Input: part model. Units: mm. Frame: model coordinates. Face numbers are marked on the shaded views. A direction names the side the tool comes from. Round coordinates to 2 decimals unless told otherwise and drop trailing zeros. Order: outer loops, then holes, each group sorted by start corner. A loop starts at its lowest first (then second) coordinate and runs counter-clockwise, first axis right, second up. Notation, with made-up numbers: (-8.75, 23) - (40.25, 23) arc R27 ccw to (40.25, 53) - close; hole circle Ø3 at (-22.75, 46.25). An arc over 180 degrees is marked (long way). One line per item, written item: value. Start each with the question number.
from build123d import *

# Parameters (mm, degrees)
SKETCH_1_W          = 67
SKETCH_1_H          = 122
EXTRUDE_1_DEPTH     = 4
SKETCH_2_W          = 4
SKETCH_2_H          = 122
EXTRUDE_2_DEPTH     = 61
FILLET_1_R          = 2
SKETCH_4_R          = 38
SKETCH_4_R_2        = 2
CUT_EXTRUDE_1_DEPTH = 11
CUT_EXTRUDE_START   = -11
SKETCH_5_R          = 36
SKETCH_5_R_2        = 2
CUT_EXTRUDE_2_DEPTH = 11


with BuildPart() as part:
    # Эскиз1 → Бобышка-Вытянуть1 (new body)
    with BuildSketch(Plane(origin=(0, 0, 0), x_dir=(1, 0, 0), z_dir=(0, 1, 0))):
        Rectangle(SKETCH_1_W, SKETCH_1_H)
    extrude(amount=EXTRUDE_1_DEPTH)

    # Эскиз2 → Бобышка-Вытянуть2 (add)
    with BuildSketch(Plane(origin=(0, 4, 0), x_dir=(1, 0, 0), z_dir=(0, 1, 0))):
        with Locations((-31.5, 0)):
            Rectangle(SKETCH_2_W, SKETCH_2_H)
        with Locations((31.5, 0)):
            Rectangle(SKETCH_2_W, SKETCH_2_H)
    extrude(amount=EXTRUDE_2_DEPTH)

    # Скругление1
    fillet_1_edges = [part.edges().sort_by_distance(p)[0] for p in [
        (-29.5, 4, 0),
        (29.5, 4, 0),
        (33.5, 0, 0),
        (-33.5, 0, 0),
    ]]
    fillet(fillet_1_edges, radius=FILLET_1_R)

    # Эскиз4 → Вырез-Вытянуть1 (cut)
    with BuildSketch(Plane(origin=(33.5, 0, 0), x_dir=(0, 0, -1), z_dir=(1, 0, 0))):
        with Locations((0, 65)):
            Circle(SKETCH_4_R)
        with Locations((0, 12)):
            Circle(SKETCH_4_R_2)
        with Locations((-31.152618372, 22.122099298)):
            Circle(SKETCH_4_R_2)
        with Locations((-50.405995364, 48.622099298)):
            Circle(SKETCH_4_R_2)
        with Locations((50.405995364, 48.622099298)):
            Circle(SKETCH_4_R_2)
        with Locations((31.152618372, 22.122099298)):
            Circle(SKETCH_4_R_2)
    extrude(amount=-CUT_EXTRUDE_1_DEPTH, mode=Mode.SUBTRACT)

    # Эскиз5 → Вырез-Вытянуть2 (cut)
    with BuildSketch(Plane.ZY.offset(33.5).offset(CUT_EXTRUDE_START)):
        with Locations((0, 65)):
            Circle(SKETCH_5_R)
        with Locations(Location((0, 12, 0), (0, 0, 180))):
            Circle(SKETCH_5_R_2)
        with Locations(Location((-31.152618372, 22.122099298, 0), (0, 0, 180))):
            Circle(SKETCH_5_R_2)
        with Locations(Location((-50.405995364, 48.622099298, 0), (0, 0, 180))):
            Circle(SKETCH_5_R_2)
        with Locations(Location((50.405995364, 48.622099298, 0), (0, 0, 180))):
            Circle(SKETCH_5_R_2)
        with Locations(Location((31.152618372, 22.122099298, 0), (0, 0, 180))):
            Circle(SKETCH_5_R_2)
    extrude(amount=CUT_EXTRUDE_2_DEPTH, mode=Mode.SUBTRACT)


solid = part.part
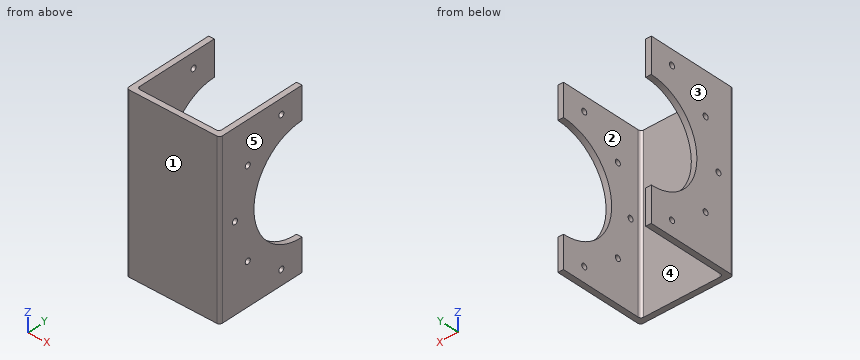
Item 1: Section query C-C on y = 38. Return loops of the section in (x, z), and give its area (3 significant figures).
Item 2: Reachability of the marked faces 4 and 5 from +Z, -Z, +X, -X, +Y, -Y: full face, straight path, thin tool, end or side. Return the list, or none.
Item 3: Section query B-B on z = 0. Return loops of the section in (x, y).
Item 4: Line query: L1, parallel to X at y = 19, z = 0.5; L2, parallel to Y at x = 31, z = 0; L3, parallel to X at y = 61, z = 36. Output: solid intervals per line, ascending.
Item 5: Section query D-D on x = -5.5. Return loops of the section in (y, z), and give its area (3 significant figures).
Item 6: Pull-direction query (X, two-part tool) for the marked faces 1, 2 and 3; classes: released by +X, released by -X, zero draft, split by the parting line, or undercut.
Item 7: First-contact query: pin 1 Ø2 at (x, z) = (4, 48.5) entering from +Y. Flat tip, straight axial feed; report the tip coordinate or a pass-through.
Item 8: Section query A-A on y = 12. Return loops of the section in (x, z), and give its area (3 significant figures).
Geometry results:
1. outline: (-33.5, -61) - (-29.5, -61) - (-29.5, -23.81) - (-33.5, -23.81) - close; (-33.5, 23.81) - (-29.5, 23.81) - (-29.5, 61) - (-33.5, 61) - close; (29.5, -61) - (33.5, -61) - (33.5, -26.74) - (29.5, -26.74) - close; (29.5, 26.74) - (33.5, 26.74) - (33.5, 61) - (29.5, 61) - close
1. area: 572 mm^2
2. face 4: +Z, -Z, +Y
2. face 5: +Z, -Z, +X, +Y, -Y
3. outline: (-33.5, 2) arc R2 ccw to (-31.5, 0) - (31.5, 0) arc R2 ccw to (33.5, 2) - (33.5, 10) - (29.5, 10) - (29.5, 6) arc R2 cw to (27.5, 4) - (-27.5, 4) arc R2 cw to (-29.5, 6) - (-29.5, 10) - (-33.5, 10) - close; (-33.5, 14) - (-29.5, 14) - (-29.5, 29) - (-33.5, 29) - close; (29.5, 14) - (33.5, 14) - (33.5, 27) - (29.5, 27) - close
4. L1: x = -33.5 to -29.5, 29.5 to 33.5
4. L2: y = 0 to 10, 14 to 27
4. L3: x = -33.5 to -29.5
5. outline: (0, -61) - (4, -61) - (4, 61) - (0, 61) - close
5. area: 488 mm^2
6. face 1: zero draft
6. face 2: undercut
6. face 3: released by -X
7. pin 1: stops at y = 4
8. outline: (-33.5, -61) - (-29.5, -61) - (-29.5, -2) - (-33.5, -2) - close; (-33.5, 2) - (-29.5, 2) - (-29.5, 61) - (-33.5, 61) - close; (29.5, -61) - (33.5, -61) - (33.5, -2) - (29.5, -2) - close; (29.5, 2) - (33.5, 2) - (33.5, 61) - (29.5, 61) - close
8. area: 944 mm^2
